Check sheet for the modelled part. Datum: model origin and axes. Units: mm. A direction names the side the tool comes from. Round coordinates to 2 decimals unless told otherwise and drop trailing zeros. Write each loop counter-clockwise with the first axis right and the second up, starting at its lowest first coordinate (ties: lowest second). Pieces come first, ordered by that corner, then holes. Notation, with made-up numbers: M 85.25,-10.75 L 142.25,-10.75 A32 cw 142.25,22.25 Z; hole C 76.5,-16 d4. An arc over 180 degrees is marked long. One line per item, written item: value.
Autodesk Inventor part; units mm, degrees
ref_plane "YZ Plane" through (0, 0, 0) normal (1, 0, 0) x (0, 1, 0)
ref_plane "XZ Plane" through (0, 0, 0) normal (0, 1, 0) x (-1, 0, 0)
ref_plane "XY Plane" through (0, 0, 0) normal (0, 0, 1) x (1, 0, 0)
sketch "Sketch1" plane through (0, 0, 0) normal (1, 0, 0) x (0, 1, 0)
  line L0 (0, 0) -> (14, 0) construction
  line L1 (14, 0) -> (14, 250)
  line L2 (14, 250) -> (0, 250) construction
  line L3 (0, 250) -> (0, 0)
  line L4 (-50, -25) -> (64, -25)
  line L5 (79, 275) -> (-65, 275)
  line L6 (8.375, 200) -> (5.625, 200)
  line L7 (5.625, 200) -> (5.625, 170)
  line L8 (5.625, 170) -> (8.375, 170)
  line L9 (8.375, 170) -> (8.375, 200)
  line L10 (8.375, 140) -> (5.625, 140)
  line L11 (5.625, 140) -> (5.625, 110)
  line L12 (5.625, 110) -> (8.375, 110)
  line L13 (8.375, 110) -> (8.375, 140)
  line L14 (8.375, 80) -> (5.625, 80)
  line L15 (5.625, 80) -> (5.625, 50)
  line L16 (5.625, 50) -> (8.375, 50)
  line L17 (8.375, 50) -> (8.375, 80)
  line L18 (8.375, 20) -> (5.625, 20)
  line L19 (5.625, 20) -> (5.625, -10)
  line L20 (5.625, -10) -> (8.375, -10)
  line L21 (8.375, -10) -> (8.375, 20)
  line L22 (8.375, 230) -> (5.625, 230)
  line L23 (5.625, 230) -> (5.625, 260)
  line L24 (5.625, 260) -> (8.375, 260)
  line L25 (8.375, 260) -> (8.375, 230)
  line L26 (-65, 275) -> (-49.85, 275)
  line L27 (-49.85, 275) -> (-49.85, 277.75)
  line L28 (-49.85, 277.75) -> (-65, 277.75)
  line L29 (-65, 277.75) -> (-65, 275)
  line L30 (79, 275) -> (63.85, 275)
  line L31 (63.85, 275) -> (63.85, 277.75)
  line L32 (63.85, 277.75) -> (79, 277.75)
  line L33 (79, 277.75) -> (79, 275)
  line L34 (-34.85, 275) -> (-19.7, 275)
  line L35 (-19.7, 275) -> (-19.7, 277.75)
  line L36 (-19.7, 277.75) -> (-34.85, 277.75)
  line L37 (-34.85, 277.75) -> (-34.85, 275)
  line L38 (33.7, 275) -> (48.85, 275)
  line L39 (48.85, 275) -> (48.85, 277.75)
  line L40 (48.85, 277.75) -> (33.7, 277.75)
  line L41 (33.7, 277.75) -> (33.7, 275)
  line L42 (-50, -25) -> (-31.85, -25)
  line L43 (-31.85, -25) -> (-31.85, -27.75)
  line L44 (-31.85, -27.75) -> (-50, -27.75)
  line L45 (-50, -27.75) -> (-50, -25)
  line L46 (-16.85, -25) -> (1.3, -25)
  line L47 (1.3, -25) -> (1.3, -27.75)
  line L48 (1.3, -27.75) -> (-16.85, -27.75)
  line L49 (-16.85, -27.75) -> (-16.85, -25)
  line L50 (12.7, -25) -> (30.85, -25)
  line L51 (30.85, -25) -> (30.85, -27.75)
  line L52 (30.85, -27.75) -> (12.7, -27.75)
  line L53 (12.7, -27.75) -> (12.7, -25)
  line L54 (64, -25) -> (45.85, -25)
  line L55 (45.85, -25) -> (45.85, -27.75)
  line L56 (45.85, -27.75) -> (64, -27.75)
  line L57 (64, -27.75) -> (64, -25)
  line L58 (0, 250) -> (-67, 275)
  line L59 (-67, 275) -> (-65, 275)
  line L60 (79, 275) -> (81, 275)
  line L61 (81, 275) -> (14, 250)
  line L62 (-50, -25) -> (-52, -25)
  line L63 (-52, -25) -> (0, 0)
  line L64 (64, -25) -> (66, -25)
  line L65 (66, -25) -> (14, 0)
  point P0 (7, 170)
  dimension "d3" = 30
  dimension "d4" = 60
  dimension "d5" = 60
  dimension "d6" = 60
  dimension "d7" = 7
  dimension "d8" = 7
  dimension "d9" = 2.75
  dimension "d10" = 15
  dimension "d11" = 50
  dimension "d12" = 50
  dimension "d13" = 25
  dimension "d14" = 25
  dimension "d15" = 65
  dimension "d16" = 300
  dimension "d17" = 65
  dimension "d18" = 60
  dimension "d19" = 2.75
  dimension "d21" = 15.15
  dimension "d22" = 15
  dimension "d24" = 15
  dimension "d27" = 2.75
  dimension "d28" = 18.15
  dimension "d29" = 15
  dimension "d30" = 15
  dimension "d31" = 11.4
  dimension "d32" = 30.15
  dimension "d34" = 68.55
  dimension "d35" = 30.15
  dimension "d44" = 2
  dimension "d45" = 2
  dimension "d46" = 2
  dimension "d47" = 2
extrude "Extrusion1" add sketch "Sketch1" along normal blind 2.75
sketch "Sketch2" plane through (0, 0, 0) normal (-1, 0, 0) x (0, 0, 1)
  line L0 (250, 0) -> (0, 0)
  line L1 (165.55, 0) -> (154.55, -11)
  line L2 (154.55, -11) -> (151.55, -11)
  line L3 (151.55, -11) -> (151.55, -3)
  line L4 (151.55, -3) -> (147.25, -3)
  line L5 (147.25, -3) -> (147.25, -11)
  line L6 (147.25, -11) -> (144.25, -11)
  line L7 (144.25, -11) -> (133.25, 0)
  line L8 (-27.75, -50) -> (-27.75, -31.85)
  dimension "d36" = 8
  dimension "d38" = 4.3
  dimension "d39" = 11
  dimension "d40" = 45
  dimension "d41" = 3
  dimension "d48" = 175
extrude "Extrusion2" add sketch "Sketch2" against normal up to surface (2.75 mm away)
equation "\"d5\" = d4"
equation "\"d6\" = d4"
equation "\"d18\" = d4"
equation "\"d30\" = d29"
properties part number "TrayPanelF"
Q1. Draft check along Z on faces 4 (the flat face through (1.356, -33.031, 262.325)), 5 (the flat face through (1.356, 47.969, 262.675)), 6 (the flat face through (0, 1, 137)). Enter one of: pulls with the +Z half, pulls with the -Z half, needs draft (parallel to the pull), parting line crosses it, or undercut.
Completed:
face 4: undercut
face 5: undercut
face 6: needs draft
Q2. Sectioned sample at B-B on y = 41.5. Enter the section's corners in (x, z), and give its area (3 significant figures).
Completed:
outline: M 0,-25 L 2.75,-25 L 2.75,-13.22 L 0,-13.22 Z; M 0,260.26 L 2.75,260.26 L 2.75,277.75 L 0,277.75 Z
area: 80.5 mm^2
Q3. Sectioned sample at D-D on z = 222. Enter the section's corners in (x, y).
Completed:
outline: M 0,0 L 2.75,0 L 2.75,14 L 0,14 Z
Q4. Sectioned sample at A-A on z = 3. Enter the section's corners in (x, y) (3 decimals).
Completed:
outline: M 0,0 L 2.75,0 L 2.75,5.625 L 0,5.625 Z; M 0,8.375 L 2.75,8.375 L 2.75,14 L 0,14 Z
Q5. Access from +Z, -Z, +X, -X, +Y, -Y to the whole of each face (thin tool, end or side, straight path). Record for faces 1 (the flat face through (1.36, -5.42, 160.13)), 2 (the flat face through (2.75, 1, 137)), 3 (the flat face through (1.356, 40.364, -12.675)).
Completed:
face 1: +X, -X, -Y
face 2: +Z, -Z, +X, +Y, -Y
face 3: +X, -X, +Y
Q6. Depth check by flat-ended pin: P1, Ø0.8, axis at x = 1, z = 58, coming from the +Y side; P2, Ø1.5, axis at x = 2, z = 139, coming from the -Y side; P3, Ø0.8, axis at x = 1, z = 276, coming from the -Y side. Enter the tip coordinate at first touch or a pass-through.
Completed:
P1: y = 14
P2: y = -6.5
P3: y = -65
Q7. Sectioned sample at C-C on x = 1. State how many separate pieces and enclosed holes the cut face has, and give its area (3 significant figures).
Completed:
separate pieces: 1
enclosed holes: 5
area: 7,330 mm^2
Q8. Scan lines: line 1 (Z direction, x = 1.6, y = 6.5); line 2 (Y direction, x = 1.95, z = 247.5) (3 decimals); line 3 (Z direction, x = 1, y = 9). Record each from-to range of solid material in increasing order. Write a range as [from, to].
Completed:
line 1: [-25, -10], [20, 50], [80, 110], [140, 170], [200, 230], [260, 275]
line 2: [0, 5.625], [8.375, 14]
line 3: [-25, 275]
